```python
from build123d import *

# Parameters (mm, degrees)
SKETCH1_W           = 13.5
SKETCH1_H           = 15.5
SKETCH1_W_2         = 11.5
SKETCH1_H_2         = 13.5
BOSS_EXTRUDE1_DEPTH = 1
BOSS_EXTRUDE2_DEPTH = 10.75
SKETCH3_W           = 3
SKETCH3_H           = 1
CUT_EXTRUDE1_DEPTH  = 5
SKETCH4_R           = 1.75
BOSS_EXTRUDE3_DEPTH = 11.75
FILLET1_R           = 1
SKETCH5_W           = 1
SKETCH5_H           = 13.5
BOSS_EXTRUDE4_DEPTH = 6
SKETCH6_W           = 1.5
SKETCH6_H           = 2.5
BOSS_EXTRUDE5_DEPTH = 5.75


with BuildPart() as part:
    # Sketch1 → Boss-Extrude1 (new body)
    # profile 1 of 2: a face of its own
    with BuildSketch(Plane(origin=(0, 0, 0), x_dir=(1, 0, 0), z_dir=(0, 1, 0))):
        Rectangle(SKETCH1_W, SKETCH1_H)
        Rectangle(SKETCH1_W_2, SKETCH1_H_2, mode=Mode.SUBTRACT)
    # profile 2 of 2: a face of its own
    with BuildSketch(Plane(origin=(0, 0, 0), x_dir=(1, 0, 0), z_dir=(0, 1, 0))):
        Rectangle(SKETCH1_W_2, SKETCH1_H_2)
    extrude(amount=BOSS_EXTRUDE1_DEPTH)

    # Sketch2 → Boss-Extrude2 (add)
    with BuildSketch(Plane(origin=(0, 1, 0), x_dir=(1, 0, 0), z_dir=(0, 1, 0))):
        Polygon((-6.75, -7.75), (6.75, -7.75), (6.75, -6.75), (5.75, -6.75), (-5.75, -6.75), (-5.75, 6.75), (5.75, 6.75), (5.75, 4.25), (6.75, 4.25), (6.75, 7.75), (-6.75, 7.75), align=None)
    extrude(amount=BOSS_EXTRUDE2_DEPTH)

    # Sketch3 → Cut-Extrude1 (cut)
    with BuildSketch(Plane(origin=(0, 11.75, 0), x_dir=(1, 0, 0), z_dir=(0, 1, 0))):
        with Locations((4.25, 7.25)):
            Rectangle(SKETCH3_W, SKETCH3_H)
    extrude(amount=-CUT_EXTRUDE1_DEPTH, mode=Mode.SUBTRACT)

    # Sketch4 → Boss-Extrude3 (add)
    # profile 1 of 6: a face of its own
    with BuildSketch(Plane(origin=(0, 11.75, 0), x_dir=(1, 0, 0), z_dir=(0, 1, 0))):
        with BuildLine():
            ThreePointArc((2.75, 10), (0, 12.75), (-2.75, 10))
            ThreePointArc((-2.75, 10), (-2.440351592, 8.732252348), (-1.58113883, 7.75))
            Line((-1.58113883, 7.75), (1.58113883, 7.75))
            ThreePointArc((1.58113883, 7.75), (2.440351592, 8.732252348), (2.75, 10))
        make_face()
        with Locations(Location((0, 10, 0), (0, 0, 270))):
            Circle(SKETCH4_R, mode=Mode.SUBTRACT)
    # profile 2 of 6: a face of its own
    with BuildSketch(Plane(origin=(0, 11.75, 0), x_dir=(1, 0, 0), z_dir=(0, 1, 0))):
        with BuildLine():
            ThreePointArc((-1.58113883, 7.75), (-2.440351592, 8.732252348), (-2.75, 10))
            Line((-2.75, 10), (-2.75, 7.75))
            Line((-2.75, 7.75), (-1.58113883, 7.75))
        make_face()
    # profile 3 of 6: a face of its own
    with BuildSketch(Plane(origin=(0, 11.75, 0), x_dir=(1, 0, 0), z_dir=(0, 1, 0))):
        with BuildLine():
            Line((2.75, 7.75), (2.75, 10))
            ThreePointArc((2.75, 10), (2.440351592, 8.732252348), (1.58113883, 7.75))
            Line((1.58113883, 7.75), (2.75, 7.75))
        make_face()
    # profile 4 of 6: a face of its own
    with BuildSketch(Plane(origin=(0, 11.75, 0), x_dir=(1, 0, 0), z_dir=(0, 1, 0))):
        with BuildLine():
            Line((-2.75, -7.75), (-2.75, -10))
            ThreePointArc((-2.75, -10), (-2.440351592, -8.732252348), (-1.58113883, -7.75))
            Line((-1.58113883, -7.75), (-2.75, -7.75))
        make_face()
    # profile 5 of 6: a face of its own
    with BuildSketch(Plane(origin=(0, 11.75, 0), x_dir=(1, 0, 0), z_dir=(0, 1, 0))):
        with BuildLine():
            ThreePointArc((-1.58113883, -7.75), (-2.440351592, -8.732252348), (-2.75, -10))
            ThreePointArc((-2.75, -10), (0, -12.75), (2.75, -10))
            ThreePointArc((2.75, -10), (2.440351592, -8.732252348), (1.58113883, -7.75))
            Line((1.58113883, -7.75), (-1.58113883, -7.75))
        make_face()
        with Locations(Location((0, -10, 0), (0, 0, 270))):
            Circle(SKETCH4_R, mode=Mode.SUBTRACT)
    # profile 6 of 6: a face of its own
    with BuildSketch(Plane(origin=(0, 11.75, 0), x_dir=(1, 0, 0), z_dir=(0, 1, 0))):
        with BuildLine():
            ThreePointArc((1.58113883, -7.75), (2.440351592, -8.732252348), (2.75, -10))
            Line((2.75, -10), (2.75, -7.75))
            Line((2.75, -7.75), (1.58113883, -7.75))
        make_face()
    extrude(amount=-BOSS_EXTRUDE3_DEPTH)

    # Fillet1
    fillet1_edges = [part.edges().sort_by_distance(p)[0] for p in [
        (-2.75, 5.875, -7.75),
        (2.75, 3.375, -7.75),
        (-2.75, 5.875, 7.75),
        (2.75, 5.875, 7.75),
        (-6.75, 5.875, 7.75),
        (-6.75, 5.875, -7.75),
        (6.75, 5.875, -7.75),
    ]]
    fillet(fillet1_edges, radius=FILLET1_R)

    # Sketch5 → Boss-Extrude4 (add)
    with BuildSketch(Plane(origin=(0, 1, 0), x_dir=(1, 0, 0), z_dir=(0, 1, 0))):
        with Locations((-5.25, 0)):
            Rectangle(SKETCH5_W, SKETCH5_H)
    extrude(amount=BOSS_EXTRUDE4_DEPTH)

    # Sketch6 → Boss-Extrude5 (add)
    with BuildSketch(Plane(origin=(0, 1, 0), x_dir=(1, 0, 0), z_dir=(0, 1, 0))):
        with Locations((5, 5.5)):
            Rectangle(SKETCH6_W, SKETCH6_H)
    extrude(amount=BOSS_EXTRUDE5_DEPTH)


solid = part.part
```
Check sheet for the modelled part. Datum: model origin and axes. Units: mm. A direction names the side the tool comes from. Give positions to 0.01 mm unless a question says otherwise; leave off trailing zeros. Loops run counter-clockwise (first coordinate to the right, second up) from the corner with the lowest first, then second, coordinate; pieces in that order, holes last. Notation, with made-up numbers: (23, -7) - (37, -7) arc R13 cw to (37, 8) - close; hole circle Ø4 at (-29, 25.5). An arc over 180 degrees is marked (long way). One line per question, with ' | ' between items. Start each with the question number.
1. Cross-section at D-D, the plane y = 6.5. Enter the section's corners in (x, z), plus the area to 3 significant figures.
2. Draft check along Z on faces 1 (the cylindrical face through (-6.465, 5.793, -7.449)), 2 (the cylindrical face through (3.051, 5.793, 8.035)), 3 (the flat face through (-6, 11.75, 1)), 4 (the flat face through (1, 1, 0)). Enter one of: released by +Z, released by -Z, zero draft, split by the parting line, or undercut.
3. Gauge pin test, flat ends, axial feed: pin 1 Ø5 at (y, z) = (5, 2.5) entering from +X; pin 2 Ø0.8 at (x, y) = (5.5, 6) entering from +Z; pin 3 Ø2.5 at (y, z) = (7, -8.5) entering from +X. Record the tip position at first contact, or that the pin passes through.
4. Set-up check for faces 5 (the flat face through (6, 5, -4.25)), 6 (the flat face through (-5, 6, 7.75)), 7 (the flat face through (-5.75, 9, 0)): record each of +Z, -Z, +X, -X, +Y, -Y from which the full face is reachable in a straight line by a thin tool's end or side.
5. Cross-section at B-B, the plane z = -10.5. Enter the section's corners in (x, y).
6. Cross-section at A-A, the plane y = 8. Enter the section's corners in (x, z).
7. Material ranges on line 1 along X through (y, z) = (4.75, -6.25); line 2 along Z through (x, y) = (-4.25, 6); line 3 along X through (y, z) = (5.25, 10), recorded low to high. Write a range as [from, to].
8. Cross-section at C-C, the plane x = 4. Enter the section's corners in (y, z).
Check result:
1) outline: (-6.75, -6.75) arc R1 ccw to (-5.75, -7.75) - (-3.75, -7.75) arc R1 cw to (-2.75, -8.75) - (-2.75, -10) arc R2.75 ccw to (2.75, -10) - (2.75, -8.75) arc R1 cw to (3.75, -7.75) - (5.75, -7.75) arc R1 ccw to (6.75, -6.75) - (6.75, -4.25) - (4.25, -4.25) - (4.25, -6.75) - (-4.75, -6.75) - (-4.75, 6.75) - (6.75, 6.75) - (6.75, 7.75) - (3.75, 7.75) arc R1 cw to (2.75, 8.75) - (2.75, 10) arc R2.75 ccw to (-2.75, 10) - (-2.75, 8.75) arc R1 cw to (-3.75, 7.75) - (-5.75, 7.75) arc R1 ccw to (-6.75, 6.75) - close; hole circle Ø3.5 at (0, -10); hole circle Ø3.5 at (0, 10) | area: 89.7 mm2
2) face 1: released by -Z | face 2: released by +Z | face 3: zero draft | face 4: undercut
3) pin 1: stops at x = -4.75 | pin 2: stops at z = 7.75 | pin 3: stops at x = 6.62
4) face 5: +X, +Y | face 6: +Z, -X, +Y, -Y | face 7: +Y
5) outline: (-2.7, 0) - (-1.68, 0) - (-1.68, 11.75) - (-2.7, 11.75) - close; (1.68, 0) - (2.7, 0) - (2.7, 11.75) - (1.68, 11.75) - close
6) outline: (-6.75, -6.75) arc R1 ccw to (-5.75, -7.75) - (-3.75, -7.75) arc R1 cw to (-2.75, -8.75) - (-2.75, -10) arc R2.75 ccw to (2.75, -10) - (2.75, -6.75) - (-5.75, -6.75) - (-5.75, 6.75) - (6.75, 6.75) - (6.75, 7.75) - (3.75, 7.75) arc R1 cw to (2.75, 8.75) - (2.75, 10) arc R2.75 ccw to (-2.75, 10) - (-2.75, 8.75) arc R1 cw to (-3.75, 7.75) - (-5.75, 7.75) arc R1 ccw to (-6.75, 6.75) - close; (5.75, -7.75) arc R1 ccw to (6.75, -6.75) - (6.75, -4.25) - (5.75, -4.25) - close; hole circle Ø3.5 at (0, -10); hole circle Ø3.5 at (0, 10)
7) line 1: x = [-6.75, -4.75], [4.25, 6.75] | line 2: z = [-7.75, -6.75], [6.75, 7.75] | line 3: x = [-2.75, -1.75], [1.75, 2.75]
8) outline: (0, -7.75) - (6.75, -7.75) - (6.75, -6.75) - (1, -6.75) - (1, 6.75) - (11.75, 6.75) - (11.75, 7.75) - (0, 7.75) - close
